```python
from build123d import *

# Parameters (mm, degrees)
BOSS_EXTRUDE1_DEPTH = 22.86
SKETCH3_R           = 1.5875
CUT_EXTRUDE1_DEPTH  = 136.30034598
SKETCH4_R           = 2.54
CUT_EXTRUDE2_DEPTH  = 136.30034598


with BuildPart() as part:
    # Sketch2 → Boss-Extrude1 (new body)
    with BuildSketch(Plane.XY):
        with BuildLine():
            Line((-20.32, 64.907113706), (-20.32, 7.660427971))
            Line((-20.32, 7.660427971), (-7.827723958, 1.407113706))
            Line((-7.827723958, 1.407113706), (7.827723958, 1.407113706))
            Line((7.827723958, 1.407113706), (20.32, 7.660427971))
            Line((20.32, 7.660427971), (20.32, 64.907113706))
            ThreePointArc((20.32, 64.907113706), (24.765, 69.352113706), (29.21, 64.907113706))
            Line((29.21, 64.907113706), (29.21, -115.432886294))
            ThreePointArc((29.21, -115.432886294), (24.765, -119.877886294), (20.32, -115.432886294))
            Line((20.32, -115.432886294), (20.32, -58.186200558))
            Line((20.32, -58.186200558), (7.827723958, -51.932886294))
            Line((7.827723958, -51.932886294), (-7.827723958, -51.932886294))
            Line((-7.827723958, -51.932886294), (-20.32, -58.186200558))
            Line((-20.32, -58.186200558), (-20.32, -115.432886294))
            ThreePointArc((-20.32, -115.432886294), (-24.765, -119.877886294), (-29.21, -115.432886294))
            Line((-29.21, -115.432886294), (-29.21, 64.907113706))
            ThreePointArc((-29.21, 64.907113706), (-24.765, 69.352113706), (-20.32, 64.907113706))
        make_face()
        Polygon((-17.78, -40.099060348), (-17.78, -51.529060348), (-7.881329635, -45.814060348), align=None, mode=Mode.SUBTRACT)
        Polygon((-20.32, -32.786200558), (-7.827723958, -39.039514822), (7.827723958, -39.039514822), (20.32, -32.786200558), (20.32, -17.739572029), (7.827723958, -11.486257765), (-7.827723958, -11.486257765), (-20.32, -17.739572029), align=None, mode=Mode.SUBTRACT)
        Polygon((-17.78, 1.003287761), (-7.881329635, -4.711712239), (-17.78, -10.426712239), align=None, mode=Mode.SUBTRACT)
        Polygon((17.78, -51.529060348), (7.881329635, -45.814060348), (17.78, -40.099060348), align=None, mode=Mode.SUBTRACT)
        Polygon((17.78, -10.426712239), (17.78, 1.003287761), (7.881329635, -4.711712239), align=None, mode=Mode.SUBTRACT)
    extrude(amount=BOSS_EXTRUDE1_DEPTH)

    # Sketch3 → Cut-Extrude1 (cut, through all)
    with BuildSketch(Plane.ZY.offset(29.21)):
        with Locations((11.43, -102.732886294)):
            Circle(SKETCH3_R)
    extrude(amount=-CUT_EXTRUDE1_DEPTH, mode=Mode.SUBTRACT)

    # Sketch4 → Cut-Extrude2 (cut, through all)
    with BuildSketch(Plane.ZY.offset(29.21)):
        with Locations((11.43, 59.827113706)):
            Circle(SKETCH4_R)
    extrude(amount=-CUT_EXTRUDE2_DEPTH, mode=Mode.SUBTRACT)


solid = part.part
```
Part model, mm, in its own coordinate system. A direction names the side the tool comes from. Coordinates: 2 decimals unless noted, no trailing zeros. Write each loop counter-clockwise with the first axis right and the second up, starting at its lowest first coordinate (ties: lowest second). Pieces come first, ordered by that corner, then holes.
Item 1: Slice it at A-A (y = -27). Write the cut outline in (x, z), and give its area (3 significant figures).
Item 2: Probe line 1 (Y direction, x = -24.25, z = 11.43); line 2 (X direction, y = 14, z = 12.5); line 3 (Y direction, x = -6.5, z = 21.5). List the from-to ranges inside material, lowest first.
Item 3: Slice it at B-B (x = -11.5). Write the cut outline in (y, z), and give its area (3 significant figures).
Item 4: Which spindle directions (+Z, -Z, +X, -X, +Y, -Y) get a long thin tool onto all of the face, cutting with end or side? Do faces 1 (the face through (-14.161, 4.578, 11.27)), 2 (the face through (0, -51.933, 11)), 3 (the face through (14.161, -14.657, 11.27)). Say none if no direction does.
Item 5: Slice it at C-C (z = 19). Count the separate pieces of the cut face and the enclosed holes in it, and give its area (3 significant figures).
Item 6: Slice it at D-D (y = 4). Write the cut outline in (x, z).
Item 7: Mould opens along Z. For faces 4 (the face through (-24.83, -101.16, 11.22)), 5 (the face through (-9, -39, 22.86)), 6 (the face through (12.76, -7.53, 11.27)), 7 (the face through (-24.827, 61.544, 9.558)) say: released by +Z, released by -Z, zero draft, split by the parting line, or undercut.
Item 8: Pin check, flat tips, straight feed: pin 1 (1 mm diameter, centred on x = -18, z = 13.5, fed in from +Y); pin 2 (4.5 mm diameter, centred on x = 3, z = 13.5, fed in from +Y); pin 3 (12 mm diameter, centred on x = -7.5, z = 20, fed in from +Y); pin 4 (4 mm diameter, centred on y = -102.73, z = 11.43, fed in from +X). Stop position of each tip, or through.
Results found:
1. outline: (-29.21, 0) - (-20.32, 0) - (-20.32, 22.86) - (-29.21, 22.86) - close; (20.32, 0) - (29.21, 0) - (29.21, 22.86) - (20.32, 22.86) - close
1. area: 406 mm2
2. line 1: y = -119.85 to -104.32, -101.15 to 57.29, 62.37 to 69.32
2. line 2: x = -29.21 to -20.32, 20.32 to 29.21
2. line 3: y = -51.93 to -39.04, -11.49 to 1.41
3. outline: (-53.77, 0) - (-47.9, 0) - (-47.9, 22.86) - (-53.77, 22.86) - close; (-43.72, 0) - (-37.2, 0) - (-37.2, 22.86) - (-43.72, 22.86) - close; (-13.32, 0) - (-6.8, 0) - (-6.8, 22.86) - (-13.32, 22.86) - close; (-2.62, 0) - (3.25, 0) - (3.25, 22.86) - (-2.62, 22.86) - close
3. area: 567 mm2
4. face 1: +Z, -Z, +Y
4. face 2: +Z, -Z, -Y
4. face 3: +Z, -Z
5. separate pieces: 1
5. enclosed holes: 5
5. area: 4,460 mm2
6. outline: (-29.21, 0) - (-13.01, 0) - (-13.01, 22.86) - (-29.21, 22.86) - close; (13.01, 0) - (29.21, 0) - (29.21, 22.86) - (13.01, 22.86) - close
7. face 4: undercut
7. face 5: released by +Z
7. face 6: zero draft
7. face 7: undercut
8. pin 1: stops at y = 6.75
8. pin 2: stops at y = 1.41
8. pin 3: stops at y = 4.25
8. pin 4: stops at x = 29.21
